Geometry check sheet. Reference: the model listing, model coordinates, mm. Face numbers are marked on the shaded views. Round coordinates to 2 decimals unless told otherwise and drop trailing zeros. Order: outer loops, then holes, each group sorted by start corner. A loop starts at its lowest first (then second) coordinate and runs counter-clockwise, first axis right, second up.
(1) Cross-section at C-C on y = -8.5. Enter the section's corners in (x, z), and give its area (3 significant figures).
(2) Gauge pin test, flat ends, axial feed: P1, Ø1, axis at x = -41, y = 1, coming from the -Z side; P2, Ø1.5, axis at x = 12, y = -0.5, coming from the +Z side; P3, Ø3, axis at y = -6, z = 47.5, coming from the +X side. Record the tip position at first contact, or that the pin passes through.
(3) Thickness scan on L1, parallel to Z at x = 0, y = 15; L2, parallel to X at y = -10.5, z = -2; L3, parallel to Z at x = 11, y = 10. Record the ranges inside material, lowest first.
(4) Cross-section at B-B on x = 0. Enter the section's corners in (y, z) (3 decimals), and give its area (3 significant figures).
(5) Draft check along Z on the marked faces 1, 2 and 3. Enter one of: pulls with the +Z half, pulls with the -Z half, needs draft (parallel to the pull), parting line crosses it, or undercut.
(6) Cross-section at A-A on z = 0. Enter the section's corners in (x, y) (3 decimals), and give its area (3 significant figures).
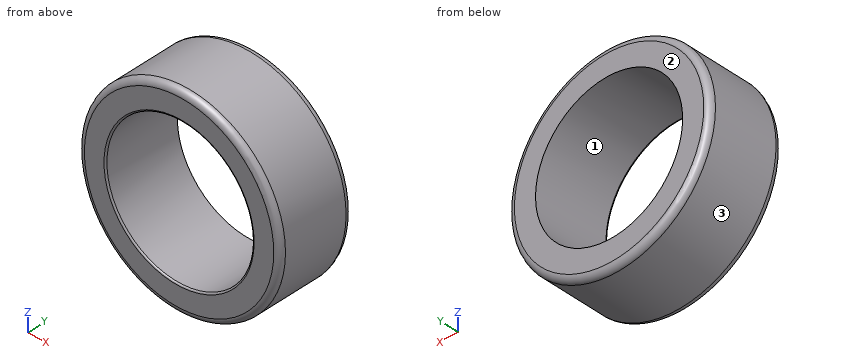
from build123d import *

# Parameters (mm, degrees)
F0_R     = 83.9597
F1_DEPTH = 32.385
F2_R     = 61.2902
F3_DEPTH = 50.8
F4_R     = 5.08
F5_R     = 1.27


with BuildPart() as f1:
    # F0 (on Front) → F1 (new body, symmetric)
    with BuildSketch(Plane.XZ):
        Circle(F0_R)
    extrude(amount=F1_DEPTH, both=True)

    # F2 (on Front) → F3 (cut, symmetric)
    with BuildSketch(Plane.XZ):
        Circle(F2_R)
    extrude(amount=F3_DEPTH, both=True, mode=Mode.SUBTRACT)

    # F4
    f4_edges = [f1.edges().sort_by_distance(p)[0] for p in [
        (-83.9597, -32.385, 0),
        (-83.9597, 32.385, 0),
    ]]
    fillet(f4_edges, radius=F4_R)

    # F5
    f5_edges = [f1.edges().sort_by_distance(p)[0] for p in [
        (-61.2902, -32.385, 0),
    ]]
    fillet(f5_edges, radius=F5_R)


solid = f1.part
Found:
1. outline: circle Ø167.92 at (0, 0); hole circle Ø122.58 at (0, 0)
1. area: 10,300 mm2
2. P1: stops at z = -73.55
2. P2: stops at z = 83.2
2. P3: stops at x = 70.24
3. L1: z = -83.96 to -61.29, 61.29 to 83.96
3. L2: x = -83.94 to -61.26, 61.26 to 83.94
3. L3: z = -83.24 to -60.3, 60.3 to 83.24
4. outline: (-32.385, -78.88) arc R5.08 ccw to (-27.305, -83.96) - (27.305, -83.96) arc R5.08 ccw to (32.385, -78.88) - (32.385, -61.29) - (-31.115, -61.29) arc R1.27 ccw to (-32.385, -62.56) - close; (-32.385, 62.56) arc R1.27 ccw to (-31.115, 61.29) - (32.385, 61.29) - (32.385, 78.88) arc R5.08 ccw to (27.305, 83.96) - (-27.305, 83.96) arc R5.08 ccw to (-32.385, 78.88) - close
4. area: 2,910 mm2
5. face 1: undercut
5. face 2: needs draft
5. face 3: parting line crosses it
6. outline: (-83.96, -27.305) arc R5.08 ccw to (-78.88, -32.385) - (-62.56, -32.385) arc R1.27 ccw to (-61.29, -31.115) - (-61.29, 32.385) - (-78.88, 32.385) arc R5.08 ccw to (-83.96, 27.305) - close; (61.29, -31.115) arc R1.27 ccw to (62.56, -32.385) - (78.88, -32.385) arc R5.08 ccw to (83.96, -27.305) - (83.96, 27.305) arc R5.08 ccw to (78.88, 32.385) - (61.29, 32.385) - close
6. area: 2,910 mm2
